Work out the finished part from the listing and answer in its coordinate system (mm). A direction names the side the tool comes from. Coordinates: 2 decimals unless noted, no trailing zeros. Order: outer loops, then holes, each group sorted by start corner. A loop starts at its lowest first (then second) coordinate and runs counter-clockwise, first axis right, second up.
```python
from build123d import *

# Parameters (mm, degrees)
F0_W          = 100
F0_H          = 100
F1_DEPTH      = 20
F2_R          = 21
F3_DEPTH      = 48
F4_R          = 21
F5_R          = 10
F6_DEPTH      = 41
F7_R          = 21
F8_DEPTH      = 53.5
F8_DEPTH_BACK = 18
F9_R          = 10
F10_W         = 60
F10_H         = 60
F11_DEPTH     = 15
F12_W         = 90
F12_H         = 90
F13_DEPTH     = 3
F15_D         = 4.2
F15_DEPTH     = 10
F15_TIP       = 1.2618073
F17_D         = 7.8
F18_R         = 3


with BuildPart() as f1:
    # F0 (on Top) → F1 (new body)
    with BuildSketch(Plane.XY):
        Rectangle(F0_W, F0_H)
    extrude(amount=F1_DEPTH)

    # F2 (on face) → F3 (join)
    with BuildSketch(Plane.XY.offset(20)):
        Circle(F2_R)
    extrude(amount=F3_DEPTH)

    # F4
    f4_edges = [f1.edges().sort_by_distance(p)[0] for p in [
        (-21, 0, 68),
    ]]
    fillet(f4_edges, radius=F4_R)

    # F5 (on Front) → F6 (join)
    with BuildSketch(Plane.XZ):
        with Locations((0, 47)):
            Circle(F5_R)
    extrude(amount=F6_DEPTH)

    # F7 (on face) → F8 (join, two sides)
    with BuildSketch(Plane.XZ.offset(41)) as f8_sk:
        with Locations((0, 47)):
            Circle(F7_R)
    extrude(amount=F8_DEPTH)
    extrude(f8_sk.sketch, amount=-F8_DEPTH_BACK)

    # F9
    f9_edges = [f1.edges().sort_by_distance(p)[0] for p in [
        (-21, -23, 47),
    ]]
    fillet(f9_edges, radius=F9_R)

    # F10 (on face) → F11 (join)
    with BuildSketch(Plane.XZ.offset(94.5)):
        with Locations((0, 47)):
            Rectangle(F10_W, F10_H)
    extrude(amount=-F11_DEPTH)

    # F12 (on face) → F13 (join)
    with BuildSketch(Plane.XZ.offset(94.5)):
        with Locations((0, 47)):
            Rectangle(F12_W, F12_H)
    extrude(amount=-F13_DEPTH)

    # F15
    with Locations(Plane.XZ.offset(94.5)):
        with Locations((-37.5, 84.5), (37.5, 84.5), (37.5, 9.5), (-37.5, 9.5)):
            Hole(F15_D / 2, depth=F15_DEPTH)
            with Locations((0, 0, -(F15_DEPTH + F15_TIP / 2))):  # 118° drill point
                Cone(0, F15_D / 2, F15_TIP, mode=Mode.SUBTRACT)

    # F17 (through all)
    with Locations(Plane(origin=(0, 0, 0), x_dir=(1, 0, 0), z_dir=(0, 0, -1))):
        with Locations((-30, 30), (30, 30), (30, -30), (-30, -30)):
            Hole(F17_D / 2)

    # F18
    f18_edges = [f1.edges().sort_by_distance(p)[0] for p in [
        (-50, -50, 10),
        (-50, 50, 10),
        (50, 50, 10),
        (50, -50, 10),
        (30, -85.5, 17),
        (45, -93, 2),
        (-30, -85.5, 17),
        (-45, -93, 2),
        (-30, -85.5, 77),
        (-45, -93, 92),
        (30, -85.5, 77),
        (45, -93, 92),
    ]]
    fillet(f18_edges, radius=F18_R)


solid = f1.part
```
1. For faces 1 (the cylindrical face through (-29.14, -85.42, 17.9)), 2 (the flat face through (-1, -91.5, 78)), 3 (the flat face through (0, -86, 77)), 4 (the flat face through (-30, -86, 47)), determine the directions among +Z, -Z, +X, -X, +Y, -Y from which every point of the face is accessible in a straight line to the end or side of a thin tool.
2. The part is cut by section D-D (y = 0). Determine the outline of the cut face in (x, z), plus the area to 3 significant figures.
3. Flat-ended cylindrical pins translate along their axes: pin 1 (17.5 mm diameter, centred on x = -1, z = 44.5, fed in from +Y); pin 2 (7 mm diameter, centred on x = 30, y = 30, fed in from -Z); pin 3 (3.5 mm diameter, centred on x = -20.5, y = -92.5, fed in from -Z); pin 4 (10 mm diameter, centred on y = -62, z = 26.5, fed in from +X). Find the tip coordinate at first contact, or state that the pin passes through.
4. The mould has two halves that part along Z. Classify faces 5 (the cylindrical face through (11.3, -56.6, 64.7)), 6 (the cylindrical face through (-1.302, -20.701, 56.915)), 7 (the flat face through (0, -86, 17)), 8 (the flat face through (-1, -94.5, 48)): released by +Z, released by -Z, zero draft, split by the parting line, or undercut.
5. Consider probe 1 along Y at (x, z) = (-30, 10); probe 2 along X at (y, z) = (30, 8); probe 3 along Z at (x, y) = (-37, -92). Determine where each line is inside the solid, lowest interval first.
6. The part is cut by section A-A (x = -37.5). Determine the outline of the cut face in (y, z).
7. The part is cut by section C-C (y = -30). Determine the outline of the cut face in (x, z), plus the area to 3 significant figures.
8. The part is cut by section B-B (x = 0). Determine the outline of the cut face in (y, z).
Worked out:
1. face 1: -Z, -X
1. face 2: none
1. face 3: +Z, +X, -X, +Y
1. face 4: +Z, -Z, -X, +Y
2. outline: (-50, 0) - (50, 0) - (50, 20) - (21, 20) - (21, 47) arc R21 ccw to (-21, 47) - (-21, 20) - (-50, 20) - close
2. area: 3,830 mm2
3. pin 1: stops at y = 21
3. pin 2: passes through
3. pin 3: stops at z = 2
3. pin 4: stops at x = 14.17
4. face 5: undercut
4. face 6: undercut
4. face 7: released by -Z
4. face 8: zero draft
5. probe 1: y = -94.5 to -91.5, -50 to -33.9, -26.1 to 26.1, 33.9 to 50
5. probe 2: x = -50 to -33.9, -26.1 to 26.1, 33.9 to 50
5. probe 3: z = 2 to 7.46, 11.54 to 82.46, 86.54 to 92
6. outline: (-94.5, 2) - (-91.5, 2) - (-91.5, 7.4) - (-94.5, 7.4) - close; (-94.5, 11.6) - (-91.5, 11.6) - (-91.5, 82.4) - (-94.5, 82.4) - close; (-94.5, 86.6) - (-91.5, 86.6) - (-91.5, 92) - (-94.5, 92) - close; (-50, 0) - (50, 0) - (50, 20) - (-50, 20) - close
7. outline: (-50, 0) - (-33.9, 0) - (-33.9, 20) - (-50, 20) - close; (-26.1, 0) - (26.1, 0) - (26.1, 20) - (-26.1, 20) - close; circle Ø41.08 at (0, 47); (33.9, 0) - (50, 0) - (50, 20) - (33.9, 20) - close
7. area: 3,010 mm2
8. outline: (-94.5, 2) - (-91.5, 2) - (-91.5, 17) - (-79.5, 17) - (-79.5, 26) - (-33, 26) arc R10 ccw to (-23, 36) - (-23, 37) - (-21, 37) - (-21, 20) - (-50, 20) - (-50, 0) - (50, 0) - (50, 20) - (21, 20) - (21, 47) arc R21 ccw to (-18.47, 57) - (-23, 57) - (-23, 58) arc R10 ccw to (-33, 68) - (-79.5, 68) - (-79.5, 77) - (-91.5, 77) - (-91.5, 92) - (-94.5, 92) - close
